Part model, mm, in its own coordinate system. A direction names the side the tool comes from. Coordinates: 2 decimals unless noted, no trailing zeros. Loops run counter-clockwise (first coordinate to the right, second up) from the corner with the lowest first, then second, coordinate; pieces in that order, holes last. Notation, with made-up numbers: M 41.25,12.25 L 90.25,12.25 A12 ccw 90.25,35.25 Z; hole C 29.5,83.25 d6. An arc over 180 degrees is marked long. Use a Markdown table: item, result. Add a question column.
1) Band-saw the part on A-A (x = 0). List the corners of the cut face in (y, z), plus the area to 4 significant figures.
2) Wall check: probe 1 along Z at (x, y) = (0, -5.25); probe 2 along Z at (x, y) = (4, -9.75); probe 3 along Y at (x, z) = (-2, -30). Give the ranges that are in metal, low to high. Write a range as from..to.
3) Band-saw the part on D-D (y = -20). List the corners of the cut face in (x, z), plus the area to 3 significant figures.
4) Tool access for faces 4 (the cylindrical face through (-28, -17, -21)), 5 (the cylindrical face through (-0.78, -2.46, 120.95)): list every direction of +Z, -Z, +X, -X, +Y, -Y with a clear straight run to the whole face (end or side of a thin tool).
5) Band-saw the part on C-C (z = -57.5). List the corners of the cut face in (x, y).
6) Pull direction Z, two halves, no side cores. Call faces 1 (the flat face through (-2, 0, 31)), 2 (the cylindrical face through (70.694, -2.465, 110.881)), 3 (the cylindrical face through (-93.87, -2.46, -55.7)): released by +Z, released by -Z, zero draft, split by the parting line, or undercut.
7) Pin check, flat tips, straight feed: pin 1 Ø14 at (x, z) = (-99.59, -57.5) entering from -Y; pin 2 Ø2 at (y, z) = (-5.5, -24.5) entering from -X; pin 3 Ø3 at (x, y) = (47, -5.5) entering from +Z. Stop position of each tip, or through.
8) Band-saw the part on B-B (z = 0). List the corners of the cut face in (x, y), plus the area to 4 significant figures.
from build123d import *

# Parameters (mm, degrees)
F0_R     = 131.5
F0_R_2   = 6
F0_R_3   = 75
F1_DEPTH = 5
F0_R_4   = 35
F2_DEPTH = 25
F0_R_5   = 30
F3_DEPTH = 10


with BuildPart() as f1:
    # F0 (on Front) → F1 (new body)
    with BuildSketch(Plane.XZ):
        Circle(F0_R)
        with Locations((-99.592921, -57.5)):
            Circle(F0_R_2, mode=Mode.SUBTRACT)
        with Locations((0, -115)):
            Circle(F0_R_2, mode=Mode.SUBTRACT)
        with Locations((99.592921, -57.5)):
            Circle(F0_R_2, mode=Mode.SUBTRACT)
        with Locations((-99.592921, 57.5)):
            Circle(F0_R_2, mode=Mode.SUBTRACT)
        Circle(F0_R_3, mode=Mode.SUBTRACT)
        with Locations((99.592921, 57.5)):
            Circle(F0_R_2, mode=Mode.SUBTRACT)
        with Locations((0, 115)):
            Circle(F0_R_2, mode=Mode.SUBTRACT)
    extrude(amount=F1_DEPTH)

    # F0 (on Front) → F2 (join)
    with BuildSketch(Plane.XZ):
        Circle(F0_R_3)
        Circle(F0_R_4, mode=Mode.SUBTRACT)
    extrude(amount=F2_DEPTH)

    # F0 (on Front) → F3 (join)
    with BuildSketch(Plane.XZ):
        Circle(F0_R_4)
        Circle(F0_R_5, mode=Mode.SUBTRACT)
    extrude(amount=F3_DEPTH)


solid = f1.part
Entries:
| question | item | result |
|---|---|---|
| 1 | outline | M -25,-75 L -5,-75 L -5,-109 L 0,-109 L 0,-30 L -10,-30 L -10,-35 L -25,-35 Z; M -25,35 L -10,35 L -10,30 L 0,30 L 0,109 L -5,109 L -5,75 L -25,75 Z; M -5,-131.5 L 0,-131.5 L 0,-121 L -5,-121 Z; M -5,121 L 0,121 L 0,131.5 L -5,131.5 Z |
| 1 | area | 2,545 mm2 |
| 2 | probe 1 | -75..-30, 30..75 |
| 2 | probe 2 | -74.89..-29.73, 29.73..74.89 |
| 2 | probe 3 | -10..0 |
| 3 | outline | C 0,0 d150; hole C 0,0 d70 |
| 3 | area | 13,800 mm2 |
| 4 | face 4 | -Y |
| 4 | face 5 | +Y, -Y |
| 5 | outline | M -118.26,-5 L -105.59,-5 L -105.59,0 L -118.26,0 Z; M -93.59,-5 L -48.15,-5 L -48.15,-25 L 48.15,-25 L 48.15,-5 L 93.59,-5 L 93.59,0 L -93.59,0 Z; M 105.59,-5 L 118.26,-5 L 118.26,0 L 105.59,0 Z |
| 6 | face 1 | zero draft |
| 6 | face 2 | split by the parting line |
| 6 | face 3 | undercut |
| 7 | pin 1 | y = -5 |
| 7 | pin 2 | x = -129.36 |
| 7 | pin 3 | z = 123.35 |
| 8 | outline | M -131.5,-5 L -75,-5 L -75,-25 L -35,-25 L -35,-10 L -30,-10 L -30,0 L -131.5,0 Z; M 30,-10 L 35,-10 L 35,-25 L 75,-25 L 75,-5 L 131.5,-5 L 131.5,0 L 30,0 Z |
| 8 | area | 2,665 mm2 |
